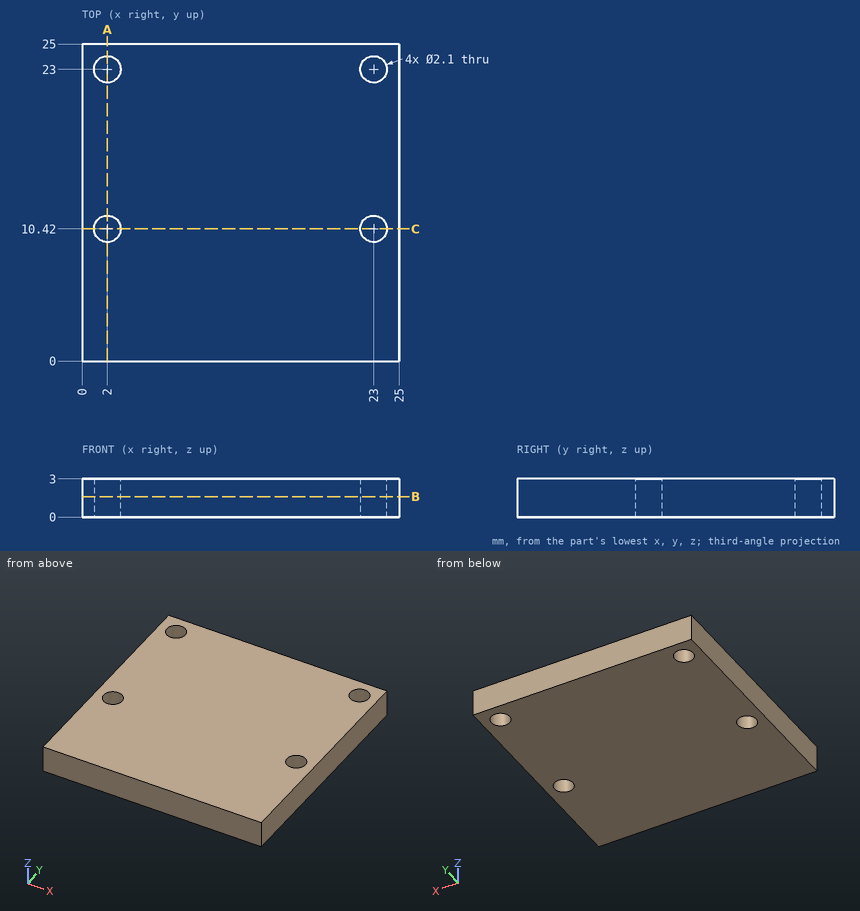
Part print with two shaded views. Sizes in mm from the minimum x, y, z corner. Coordinates: 2 decimals unless noted, no trailing zeros. Write each loop counter-clockwise with the first axis right and the second up, starting at its lowest first coordinate (ties: lowest second). Pieces come first, ordered by that corner, then holes.
(1) Cut at A-A on x = 2. List the corners of the cut face in (y, z).
(2) Cut at C-C on y = 10.42. List the corners of the cut face in (x, z), and give its area (3 significant figures).
(3) Drill centre lines: line 1 (X direction, y = 10.25, z = 2); line 2 (X direction, y = 23.75, z = 2.45). Where is each one in solid material? Low to high.
(4) Cut at B-B on z = 1.6. List the corners of the cut face in (x, y), and give its area (3 significant figures).
Working result:
1. outline: (0, 0) - (9.37, 0) - (9.37, 3) - (0, 3) - close; (11.47, 0) - (21.95, 0) - (21.95, 3) - (11.47, 3) - close; (24.05, 0) - (25, 0) - (25, 3) - (24.05, 3) - close
2. outline: (0, 0) - (0.95, 0) - (0.95, 3) - (0, 3) - close; (3.05, 0) - (21.95, 0) - (21.95, 3) - (3.05, 3) - close; (24.05, 0) - (25, 0) - (25, 3) - (24.05, 3) - close
2. area: 62.4 mm2
3. line 1: x = 0 to 0.96, 3.04 to 21.96, 24.04 to 25
3. line 2: x = 0 to 1.27, 2.73 to 22.27, 23.73 to 25
4. outline: (0, 0) - (25, 0) - (25, 25) - (0, 25) - close; hole circle Ø2.1 at (2, 10.42); hole circle Ø2.1 at (2, 23); hole circle Ø2.1 at (23, 10.42); hole circle Ø2.1 at (23, 23)
4. area: 611 mm2
